For this review, take the finished solid that the model builds, in its own axes (mm). Coordinates: 2 decimals unless noted, no trailing zeros. Write each loop counter-clockwise with the first axis right and the second up, starting at its lowest first coordinate (ties: lowest second). Pieces come first, ordered by that corner, then holes.
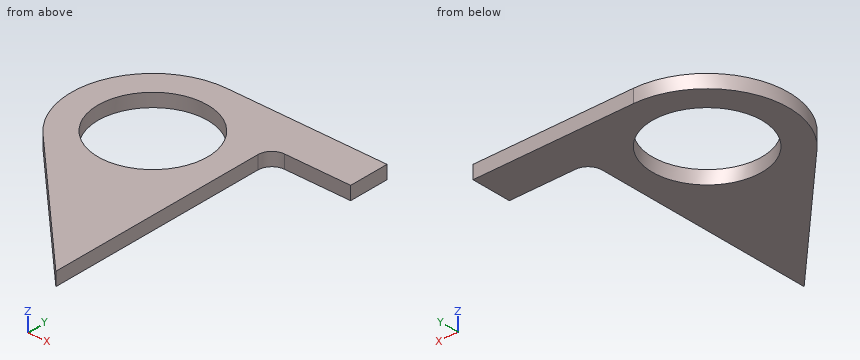
```python
from build123d import *

# Parameters (mm, degrees)
SKETCH1_R           = 26.035
BOSS_EXTRUDE1_DEPTH = 6.35
FILLET1_R           = 6.604


with BuildPart() as part:
    # Sketch1 → Boss-Extrude1 (new body)
    with BuildSketch(Plane(origin=(0, 0, 457.2), x_dir=(-1, 0, 0), z_dir=(0, 0, -1))):
        with BuildLine():
            Line((273.05, 603.25), (273.05, 584.2))
            Line((273.05, 584.2), (311.15, 584.2))
            Line((311.15, 584.2), (311.15, 471.635437661))
            Line((311.15, 471.635437661), (376.639781169, 537.125218831))
            ThreePointArc((376.639781169, 537.125218831), (385.036473692, 579.338242753), (349.25, 603.25))
            Line((349.25, 603.25), (273.05, 603.25))
        make_face()
        with Locations((349.25, 564.515)):
            Circle(SKETCH1_R, mode=Mode.SUBTRACT)
    extrude(amount=BOSS_EXTRUDE1_DEPTH)

    # Fillet1
    fillet1_edges = [part.edges().sort_by_distance(p)[0] for p in [
        (-311.15, 584.2, 454.025),
    ]]
    fillet(fillet1_edges, radius=FILLET1_R)


solid = part.part
```
Q1. Clearance check with flat-ended pins moving along their axes: pin 1 Ø2 at (y, z) = (514, 451.5) entering from -X; pin 2 Ø3 at (y, z) = (538, 453.5) entering from +X; pin 3 Ø10 at (x, y) = (-290.5, 575) entering from +Z. State where each tip first meets the part, or that it passes through.
Ans:
pin 1: stops at x = -354.51
pin 2: stops at x = -311.15
pin 3: passes through
Q2. For probe 1 along X at (y, z) = (557, 456.25); probe 2 along X at (y, z) = (547.5, 456.75); probe 3 along Y at (x, z) = (-365, 452), list the stretches that pass through material, from the lowest coordinate up.
Ans:
probe 1: x = -387.25 to -374.18, -324.32 to -311.15
probe 2: x = -384.05 to -368.96, -329.54 to -311.15
probe 3: y = 525.49 to 543.78, 585.25 to 599.9
Q3. Add section C-C (x = -352). State the section outline as (y, z) points.
Ans:
outline: (512.49, 450.85) - (538.63, 450.85) - (538.63, 457.2) - (512.49, 457.2) - close; (590.4, 450.85) - (603.15, 450.85) - (603.15, 457.2) - (590.4, 457.2) - close
Q4. Add section B-B (z = 456). State the section outline as (x, y) points (3 decimals), then the cut area to 3 significant figures.
Ans:
outline: (-376.64, 537.125) - (-311.15, 471.635) - (-311.15, 577.596) arc R6.604 cw to (-304.546, 584.2) - (-273.05, 584.2) - (-273.05, 603.25) - (-349.25, 603.25) arc R38.735 ccw to start; hole circle Ø52.07 at (-349.25, 564.515)
area: 5,410 mm2
Q5. Add section D-D (y = 592). State the section outline as (x, z) points, then the cut area to 3 significant figures.
Ans:
outline: (-376.54, 450.85) - (-273.05, 450.85) - (-273.05, 457.2) - (-376.54, 457.2) - close
area: 657 mm2
Q6. Add section A-A (x = -338). State the section outline as (y, z) points, then the cut area to 3 significant figures.
Ans:
outline: (498.49, 450.85) - (541.04, 450.85) - (541.04, 457.2) - (498.49, 457.2) - close; (587.99, 450.85) - (603.25, 450.85) - (603.25, 457.2) - (587.99, 457.2) - close
area: 367 mm2
